from build123d import *

# Parameters (mm, degrees)
CYLINDER064_R               = 4.8
CYLINDER064_DEPTH           = 18
CYLINDER064_ROLL_ANGLE      = -89.999776
CYLINDER064_PITCH_ANGLE     = 1.4e-05
CYLINDER064_PLACEMENT_ANGLE = -9.999925
PAD011_DEPTH                = 47
CYLINDER051_R               = 1.75
CYLINDER051_DEPTH           = 18
CYLINDER051_ROLL_ANGLE      = -89.999776
CYLINDER051_PITCH_ANGLE     = 1.4e-05
CYLINDER051_PLACEMENT_ANGLE = -9.999925
CYLINDER053_R               = 1.75
CYLINDER053_DEPTH           = 18
CYLINDER053_ROLL_ANGLE      = -89.999776
CYLINDER053_PITCH_ANGLE     = 1.4e-05
CYLINDER053_PLACEMENT_ANGLE = -9.999925
CYLINDER054_R               = 1.75
CYLINDER054_DEPTH           = 18
CYLINDER054_ROLL_ANGLE      = -89.999776
CYLINDER054_PITCH_ANGLE     = 1.4e-05
CYLINDER054_PLACEMENT_ANGLE = -9.999925
CYLINDER059_R               = 1.75
CYLINDER059_DEPTH           = 18
CYLINDER059_ROLL_ANGLE      = -89.999776
CYLINDER059_PITCH_ANGLE     = 1.4e-05
CYLINDER059_PLACEMENT_ANGLE = -9.999925
CYLINDER055_R               = 10
CYLINDER055_DEPTH           = 3
CYLINDER055_ROLL_ANGLE      = -89.999807
CYLINDER055_PITCH_ANGLE     = 8e-06
CYLINDER055_PLACEMENT_ANGLE = -9.999933


with BuildPart() as cylinder064:
    # Cylinder064 → Cylinder064 (new body)
    with BuildSketch(Plane.XY):
        Circle(CYLINDER064_R)
    extrude(amount=CYLINDER064_DEPTH)


with BuildPart() as cylinder064_1:
    # Cylinder064 roll: moved
    add(cylinder064.part.rotate(Axis((0, 0, 0), (1, 0, 0)), CYLINDER064_ROLL_ANGLE))


with BuildPart() as cylinder064_2:
    # Cylinder064 pitch: moved
    add(cylinder064_1.part.rotate(Axis((0, 0, 0), (0, 1, 0)), CYLINDER064_PITCH_ANGLE))


with BuildPart() as cylinder064_3:
    # Cylinder064 placement: moved
    add(cylinder064_2.part.moved(Location((35.146424, -29.285947, 16.499989))).rotate(Axis((35.146424, -29.285947, 16.499989), (0, 0, 1)), CYLINDER064_PLACEMENT_ANGLE))


with BuildPart() as winkel_p001:
    # Sketch011 → Pad011 (new body)
    with BuildSketch(Plane.XY):
        Polygon((29.25, 0), (25.25, 0), (25.25, -28), (44.946155, -31.472964), (45.640748, -27.533733), (29.25, -24.643601), align=None)
    extrude(amount=PAD011_DEPTH)


with BuildPart() as winkel_p001_1:
    # Body013 placement: moved
    add(winkel_p001.part.moved(Location((0, 0, -7))))


with BuildPart() as cylinder051:
    # Cylinder051 → Cylinder051 (new body)
    with BuildSketch(Plane.XY):
        Circle(CYLINDER051_R)
    extrude(amount=CYLINDER051_DEPTH)


with BuildPart() as cylinder051_1:
    # Cylinder051 roll: moved
    add(cylinder051.part.rotate(Axis((0, 0, 0), (1, 0, 0)), CYLINDER051_ROLL_ANGLE))


with BuildPart() as cylinder051_2:
    # Cylinder051 pitch: moved
    add(cylinder051_1.part.rotate(Axis((0, 0, 0), (0, 1, 0)), CYLINDER051_PITCH_ANGLE))


with BuildPart() as cylinder051_3:
    # Cylinder051 placement: moved
    add(cylinder051_2.part.moved(Location((32.058057, -23.765835, 25.500009))).rotate(Axis((32.058057, -23.765835, 25.500009), (0, 0, 1)), CYLINDER051_PLACEMENT_ANGLE))


with BuildPart() as cylinder053:
    # Cylinder053 → Cylinder053 (new body)
    with BuildSketch(Plane.XY):
        Circle(CYLINDER053_R)
    extrude(amount=CYLINDER053_DEPTH)


with BuildPart() as cylinder053_1:
    # Cylinder053 roll: moved
    add(cylinder053.part.rotate(Axis((0, 0, 0), (1, 0, 0)), CYLINDER053_ROLL_ANGLE))


with BuildPart() as cylinder053_2:
    # Cylinder053 pitch: moved
    add(cylinder053_1.part.rotate(Axis((0, 0, 0), (0, 1, 0)), CYLINDER053_PITCH_ANGLE))


with BuildPart() as cylinder053_3:
    # Cylinder053 placement: moved
    add(cylinder053_2.part.moved(Location((39.936521, -25.15501, 25.500007))).rotate(Axis((39.936521, -25.15501, 25.500007), (0, 0, 1)), CYLINDER053_PLACEMENT_ANGLE))


with BuildPart() as cylinder054:
    # Cylinder054 → Cylinder054 (new body)
    with BuildSketch(Plane.XY):
        Circle(CYLINDER054_R)
    extrude(amount=CYLINDER054_DEPTH)


with BuildPart() as cylinder054_1:
    # Cylinder054 roll: moved
    add(cylinder054.part.rotate(Axis((0, 0, 0), (1, 0, 0)), CYLINDER054_ROLL_ANGLE))


with BuildPart() as cylinder054_2:
    # Cylinder054 pitch: moved
    add(cylinder054_1.part.rotate(Axis((0, 0, 0), (0, 1, 0)), CYLINDER054_PITCH_ANGLE))


with BuildPart() as cylinder054_3:
    # Cylinder054 placement: moved
    add(cylinder054_2.part.moved(Location((32.055183, -23.766017, 7.500006))).rotate(Axis((32.055183, -23.766017, 7.500006), (0, 0, 1)), CYLINDER054_PLACEMENT_ANGLE))


with BuildPart() as cylinder059:
    # Cylinder059 → Cylinder059 (new body)
    with BuildSketch(Plane.XY):
        Circle(CYLINDER059_R)
    extrude(amount=CYLINDER059_DEPTH)


with BuildPart() as cylinder059_1:
    # Cylinder059 roll: moved
    add(cylinder059.part.rotate(Axis((0, 0, 0), (1, 0, 0)), CYLINDER059_ROLL_ANGLE))


with BuildPart() as cylinder059_2:
    # Cylinder059 pitch: moved
    add(cylinder059_1.part.rotate(Axis((0, 0, 0), (0, 1, 0)), CYLINDER059_PITCH_ANGLE))


with BuildPart() as cylinder059_3:
    # Cylinder059 placement: moved
    add(cylinder059_2.part.moved(Location((39.936529, -25.15494, 7.500007))).rotate(Axis((39.936529, -25.15494, 7.500007), (0, 0, 1)), CYLINDER059_PLACEMENT_ANGLE))


with BuildPart() as cut061:
    # Cylinder055 → Cylinder055 (new body)
    with BuildSketch(Plane.XY):
        Circle(CYLINDER055_R)
    extrude(amount=CYLINDER055_DEPTH)


with BuildPart() as cut061_1:
    # Cylinder055 roll: moved
    add(cut061.part.rotate(Axis((0, 0, 0), (1, 0, 0)), CYLINDER055_ROLL_ANGLE))


with BuildPart() as cut061_2:
    # Cylinder055 pitch: moved
    add(cut061_1.part.rotate(Axis((0, 0, 0), (0, 1, 0)), CYLINDER055_PITCH_ANGLE))


with BuildPart() as cut061_3:
    # Cylinder055 placement: moved
    add(cut061_2.part.moved(Location((38.083572, -12.645952, 16.50004))).rotate(Axis((38.083572, -12.645952, 16.50004), (0, 0, 1)), CYLINDER055_PLACEMENT_ANGLE))

    # Cut053: cut Cylinder059
    add(cylinder059_3.part, mode=Mode.SUBTRACT)

    # Cut054: cut Cylinder054
    add(cylinder054_3.part, mode=Mode.SUBTRACT)

    # Cut055: cut Cylinder053
    add(cylinder053_3.part, mode=Mode.SUBTRACT)

    # Cut056: cut Cylinder051
    add(cylinder051_3.part, mode=Mode.SUBTRACT)

    # Cut057: cut winkel_p001
    add(winkel_p001_1.part, mode=Mode.SUBTRACT)

    # Cut061: cut Cylinder064
    add(cylinder064_3.part, mode=Mode.SUBTRACT)


solid = cut061_3.part
The listing builds one solid part. Answer for the finished solid, in the listing's coordinates (mm). Coordinates: 2 decimals unless noted, no trailing zeros.
1) Flat-ended cylindrical pins translate along their axes: pin 1 Ø6 at (x, z) = (38, 18) entering from +Y; pin 2 Ø6 at (x, z) = (46, 14.5) entering from +Y; pin 3 Ø1.5 at (x, z) = (43, 10) entering from +Y. Find the tip coordinate at first contact, or state that the pin passes through.
2) Find the intervals of material crossed by L1, parallel to Y at x = 47, z = 14.5; L2, parallel to Y at x = 39.75, z = 12.5; L3, parallel to Z at x = 46.75, y = -12.75, in increasing order.
3) Determine the mould class of faces 1 (the face through (29.25, -10, 16)), 2 (the face through (42.54, -12.88, 18.34)), 3 (the face through (48.188, -12.926, 16.637)), 4 (the face through (30.51, -9.809, 10.435)) for opening direction Y: pulls with the +Y half, pulls with the -Y half, needs draft (parallel to the pull), parting line crosses it, or undercut.
Values:
1. pin 1: stops at y = -9.06
1. pin 2: stops at y = -10.47
1. pin 3: stops at y = -10.33
2. L1: y = -14.22 to -11.17
2. L2: y = -11.82 to -9.89
2. L3: z = 11.32 to 21.68
3. face 1: needs draft
3. face 2: undercut
3. face 3: pulls with the -Y half
3. face 4: pulls with the +Y half
